from build123d import *

# Parameters (mm, degrees)
SKETCH1_R          = 4
BASE_FLANGE1_DEPTH = 15
SKETCH6_W          = 500
SKETCH6_H          = 42
CUT_EXTRUDE1_DEPTH = 381.59689962
CHAMFER1_SIZE      = 10


# Sheet-metal steps are written as plain solids
with BuildPart() as part:
    # Sketch1 → Base-Flange1 (new body)
    with BuildSketch(Plane(origin=(0, 0, 0), x_dir=(1, 0, 0), z_dir=(0, 1, 0))):
        with BuildLine():
            Line((372, 50), (377, 50))
            Line((377, 50), (377, -50))
            Line((377, -50), (-377, -50))
            Line((-377, -50), (-377, 50))
            Line((-377, 50), (-372, 50))
            ThreePointArc((-372, 50), (-332, 10), (-292, 50))
            Line((-292, 50), (-289, 50))
            ThreePointArc((-289, 50), (-249, 10), (-209, 50))
            Line((-209, 50), (-206, 50))
            ThreePointArc((-206, 50), (-166, 10), (-126, 50))
            Line((-126, 50), (-123, 50))
            ThreePointArc((-123, 50), (-83, 10), (-43, 50))
            Line((-43, 50), (-40, 50))
            ThreePointArc((-40, 50), (0, 10), (40, 50))
            Line((40, 50), (43, 50))
            ThreePointArc((43, 50), (83, 10), (123, 50))
            Line((123, 50), (126, 50))
            ThreePointArc((126, 50), (166, 10), (206, 50))
            Line((206, 50), (209, 50))
            ThreePointArc((209, 50), (249, 10), (289, 50))
            Line((289, 50), (292, 50))
            ThreePointArc((292, 50), (332, 10), (372, 50))
        make_face()
        with Locations(Location((-320, -20, 0), (0, 0, 270))):
            Circle(SKETCH1_R, mode=Mode.SUBTRACT)
        with Locations(Location((320, -20, 0), (0, 0, 90))):
            Circle(SKETCH1_R, mode=Mode.SUBTRACT)
    extrude(amount=-BASE_FLANGE1_DEPTH)

    # Sketch6 → Cut-Extrude1 (cut, through all)
    with BuildSketch(Plane(origin=(0, 0, 0), x_dir=(1, 0, 0), z_dir=(0, 1, 0))):
        with Locations((0, -29)):
            Rectangle(SKETCH6_W, SKETCH6_H)
    extrude(amount=-CUT_EXTRUDE1_DEPTH, mode=Mode.SUBTRACT)

    # Chamfer1
    chamfer1_edges = [part.edges().sort_by_distance(p)[0] for p in [
        (377, -7.5, 50),
        (-377, -7.5, 50),
        (-250, -7.5, 50),
        (-250, -7.5, 8),
        (250, -7.5, 8),
        (250, -7.5, 50),
    ]]
    chamfer(chamfer1_edges, length=CHAMFER1_SIZE)


solid = part.part
Here's how the part is built. I have some questions about the finished solid (model axes, mm). A direction names the side the tool comes from. Round coordinates to 2 decimals unless told otherwise and drop trailing zeros. Order: outer loops, then holes, each group sorted by start corner. A loop starts at its lowest first (then second) coordinate and runs counter-clockwise, first axis right, second up. Notation, with made-up numbers: M 85.5,-28.75 L 142.5,-28.75 A11 cw 142.5,-10.75 Z; hole C 71.5,46 d3. An arc over 180 degrees is marked long. Return JSON: item names as keys, results as strings. Group by question number.
1. On a 3-axis mill with a long thin cutter (end or side, diameter ignored), from which of +Z, -Z, +X, -X, +Y, -Y can I reach the whole of each face in a straight line? I mean faces 1 (the face through (-3, -7, 8)), 2 (the face through (2, 0, 0)). Say none if no direction works.
2. Please list where these lines run through material, in increasing order: probe 1 along X at (y, z) = (-12, 20); probe 2 along X at (y, z) = (-11.5, 33.5); probe 3 along Z at (x, y) = (320, -8.75).
3. If we section it at A-A on y = -7.75: State how many separate pieces and enclosed holes the cut face has, then the cut area to 3 significant figures.
4. I'm going to push flat-ended pins straight in: pin 1 Ø4 at (x, y) = (123.5, -4) entering from +Z; pin 2 Ø3 at (x, y) = (-53, -3) entering from -Z; pin 3 Ø7 at (x, z) = (-320, 20) entering from -Y; pin 4 Ø1 at (x, y) = (-76, -2) entering from -Z. Where does each tip first touch, or does it pass through?
5. If we section it at B-B on x = 83: List the corners of the cut face in (y, z) for me, then the cut area to 3 significant figures.
6. If we mould it in two halves opening along X, with no side actions, what happens to faces 3 (the face through (-377, -7, -4)), 4 (the face through (250, -7, 29)), 5 (the face through (-313, -7, 50))? For each: pulls with the +X half, pulls with the -X half, needs draft (parallel to the pull), parting line crosses it, or undercut.
7. If we section it at D-D on x = -332: List the corners of the cut face in (y, z) for me, then the cut area to 3 significant figures.
Reply:
{
 "1": {"face 1": "+Z, +Y, -Y", "face 2": "+Z, -Z, +X, -X, +Y"},
 "2": {"probe 1": "-377 to -324, -316 to -250, 250 to 316, 324 to 377", "probe 2": "-377 to -250, 250 to 377", "probe 3": "-11.84 to 16, 24 to 50"},
 "3": {"separate pieces": "1", "enclosed holes": "2", "area": "31,600 mm^2"},
 "4": {"pin 1": "z = 8", "pin 2": "z = -25.35", "pin 3": "through", "pin 4": "z = -10.71"},
 "5": {"outline": "M -15,-10 L 0,-10 L 0,8 L -15,8 Z", "area": "270 mm^2"},
 "6": {"face 3": "pulls with the -X half", "face 4": "undercut", "face 5": "needs draft"},
 "7": {"outline": "M -15,-10 L 0,-10 L 0,50 L -15,50 Z", "area": "900 mm^2"}
}
